Model file for the job. Use its own axes, mm. Round coordinates to 2 decimals unless told otherwise and drop trailing zeros. Order: outer loops, then holes, each group sorted by start corner. A loop starts at its lowest first (then second) coordinate and runs counter-clockwise, first axis right, second up. Notation, with made-up numbers: (57.25, 85) - (111.25, 85) arc R3 cw to (111.25, 89) - close; hole circle Ø4 at (67.25, -39.5). An arc over 180 degrees is marked (long way). Answer as CSV lines item,"result". Start each with the question number.
1. Pull direction X, two halves, no side cores. Call faces 1 (the face through (1.18, -2.26, 3.04)), 2 (the face through (0, 3, 0)), 3 (the face through (-3.746, 0.165, 2.254)): released by +X, released by -X, zero draft, split by the parting line, or undercut.
2. Wall check: line 1 along Y through (x, z) = (0, 2.85); line 2 along X through (y, z) = (-1.5, 4.75); line 3 along X through (y, z) = (1, 5.4). Give the ranges that are in metal, low to high. Write a range as [from, to].
3. Band-saw the part on A-A on y = 0. List the corners of the cut face in (x, z), then the cut area to 3 significant figures.
4. Pin check, flat tips, straight feed: pin 1 Ø1.5 at (x, z) = (1.5, 2.5) entering from +Y; pin 2 Ø1.5 at (y, z) = (-0.5, 3) entering from -X; pin 3 Ø3 at (x, z) = (-2.5, 1.5) entering from -Y. Stop position of each tip, or through.
5. Band-saw the part on C-C on z = 3.6. List the corners of the cut face in (x, y).
```python
from build123d import *

# Parameters (mm, degrees)
F0_R     = 3.75
F1_DEPTH = 6
F2_R     = 2.55
F3_DEPTH = 6
F4_SIZE2 = 1.4281480067
F4_SIZE  = 1


with BuildPart() as f1:
    # F0 (on Top) → F1 (new body)
    with BuildSketch(Plane.XY):
        Circle(F0_R)
    extrude(amount=F1_DEPTH)

    # F2 (on face) → F3 (cut, through all)
    with BuildSketch(Plane.XY.offset(6)):
        Circle(F2_R)
    extrude(amount=-F3_DEPTH, mode=Mode.SUBTRACT)

    # F4
    f4_edges = [f1.edges().sort_by_distance(p)[0] for p in [
        (-3.75, 0, 6),
    ]]
    f4_side = f1.faces().sort_by_distance((-3.643934, 0, 6))[0]
    chamfer(f4_edges, length=F4_SIZE, length2=F4_SIZE2, reference=f4_side)


solid = f1.part
```
Reply:
1,face 1,"undercut"
1,face 2,"zero draft"
1,face 3,"split by the parting line"
2,line 1,"y = [-3.75, -2.55], [2.55, 3.75]"
2,line 2,"x = [-3.3, -2.06], [2.06, 3.3]"
2,line 3,"x = [-3.01, -2.35], [2.35, 3.01]"
3,outline,"(-3.75, 0) - (-2.55, 0) - (-2.55, 6) - (-2.75, 6) - (-3.75, 4.57) - close; (2.55, 0) - (3.75, 0) - (3.75, 4.57) - (2.75, 6) - (2.55, 6) - close"
3,area,"13.0 mm2"
4,pin 1,"stops at y = 3.67"
4,pin 2,"stops at x = -3.75"
4,pin 3,"stops at y = -3.61"
5,outline,"circle Ø7.5 at (0, 0); hole circle Ø5.1 at (0, 0)"
